Could you check a few things on this model? Use its own coordinates, in mm. Give positions to 0.01 mm unless a question says otherwise; leave off trailing zeros. Write each loop counter-clockwise with the first axis right and the second up, starting at its lowest first coordinate (ties: lowest second). Pieces come first, ordered by that corner, then holes. Notation, with made-up numbers: (-8.75, 9) - (13.25, 9) arc R21 cw to (13.25, 42) - close; hole circle Ø8 at (-13, -33.5). An arc over 180 degrees is marked (long way). Answer in a Markdown table with one row per item.
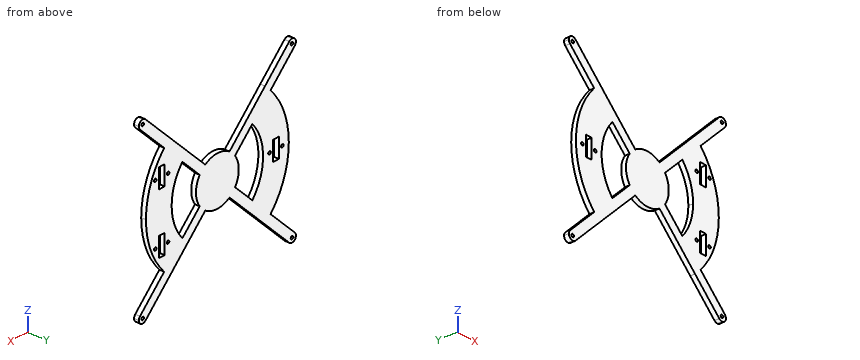
from build123d import *

# Parameters (mm, degrees)
SKETCH1_W           = 220
SKETCH1_H           = 220
SKETCH1_R           = 1.8
SKETCH1_W_2         = 8
SKETCH1_H_2         = 24
BOSS_EXTRUDE1_DEPTH = 3
CUT_EXTRUDE1_DEPTH  = 10


with BuildPart() as part:
    # Sketch1 → Boss-Extrude1 (new, symmetric)
    with BuildSketch(Plane(origin=(0, 0, 0), x_dir=(1, 0, 0), z_dir=(0, 1, 0))):
        Rectangle(SKETCH1_W, SKETCH1_H)
        with Locations(Location((-104.5, 104.5, 0), (0, 0, 270))):
            Circle(SKETCH1_R, mode=Mode.SUBTRACT)
        with Locations(Location((104.5, 104.5, 0), (0, 0, 90))):
            Circle(SKETCH1_R, mode=Mode.SUBTRACT)
        with Locations(Location((104.5, -104.5, 0), (0, 0, 270))):
            Circle(SKETCH1_R, mode=Mode.SUBTRACT)
        with Locations(Location((-104.5, -104.5, 0), (0, 0, 90))):
            Circle(SKETCH1_R, mode=Mode.SUBTRACT)
        with Locations(Location((-73, 0, 0), (0, 0, 270))):
            Circle(SKETCH1_R, mode=Mode.SUBTRACT)
        with Locations(Location((-91, 0, 0), (0, 0, 270))):
            Circle(SKETCH1_R, mode=Mode.SUBTRACT)
        with Locations(Location((87, 37, 0), (0, 0, 270))):
            Circle(SKETCH1_R, mode=Mode.SUBTRACT)
        with Locations(Location((69, 37, 0), (0, 0, 270))):
            Circle(SKETCH1_R, mode=Mode.SUBTRACT)
        with Locations(Location((87, -37, 0), (0, 0, 270))):
            Circle(SKETCH1_R, mode=Mode.SUBTRACT)
        with Locations(Location((69, -37, 0), (0, 0, 270))):
            Circle(SKETCH1_R, mode=Mode.SUBTRACT)
        with Locations((-82, 0)):
            Rectangle(SKETCH1_W_2, SKETCH1_H_2, mode=Mode.SUBTRACT)
        with Locations((78, 37)):
            Rectangle(SKETCH1_W_2, SKETCH1_H_2, mode=Mode.SUBTRACT)
        with Locations((78, -37)):
            Rectangle(SKETCH1_W_2, SKETCH1_H_2, mode=Mode.SUBTRACT)
    extrude(amount=BOSS_EXTRUDE1_DEPTH, both=True)

    # Sketch2 → Cut-Extrude1 (cut)
    with BuildSketch(Plane.XZ.offset(3)):
        with BuildLine():
            ThreePointArc((-108.389087297, 100.610912703), (-109.581337429, 102.395241122), (-110, 104.5))
            Line((-110, 104.5), (-110, -104.50000001))
            ThreePointArc((-110, -104.50000001), (-109.581337431, -102.395241127), (-108.389087297, -100.610912703))
            Line((-108.389087297, -100.610912703), (-74.492734511, -66.714559918))
            ThreePointArc((-74.492734511, -66.714559918), (-100, 0), (-74.492734511, 66.714559918))
            Line((-74.492734511, 66.714559918), (-108.389087297, 100.610912703))
        make_face()
        with BuildLine():
            Line((-24.74274405, 16.964569457), (-48.976502392, 41.198327799))
            ThreePointArc((-48.976502392, 41.198327799), (-64, 0), (-48.976502392, -41.198327799))
            Line((-48.976502392, -41.198327799), (-24.74274405, -16.964569457))
            ThreePointArc((-24.74274405, -16.964569457), (-30, 0), (-24.74274405, 16.964569457))
        make_face()
        with BuildLine():
            ThreePointArc((64, 0), (60.126933038, 21.926055812), (48.976502392, 41.198327799))
            Line((48.976502392, 41.198327799), (24.74274405, 16.964569457))
            ThreePointArc((24.74274405, 16.964569457), (28.65556073, 8.880249954), (30, 0))
            ThreePointArc((30, 0), (28.65556073, -8.880249954), (24.74274405, -16.964569457))
            Line((24.74274405, -16.964569457), (48.976502392, -41.198327799))
            ThreePointArc((48.976502392, -41.198327799), (60.126933038, -21.926055812), (64, 0))
        make_face()
        with BuildLine():
            Line((110, -104.5), (110, 104.5))
            ThreePointArc((110, 104.5), (109.581337429, 102.395241122), (108.389087297, 100.610912703))
            Line((108.389087297, 100.610912703), (74.492734511, 66.714559918))
            ThreePointArc((74.492734511, 66.714559918), (93.405763878, 35.71222864), (100, 0))
            ThreePointArc((100, 0), (93.405763878, -35.71222864), (74.492734511, -66.714559918))
            Line((74.492734511, -66.714559918), (108.389087297, -100.610912703))
            ThreePointArc((108.389087297, -100.610912703), (109.581337429, -102.395241122), (110, -104.5))
        make_face()
        with BuildLine():
            Line((-104.500000026, 110), (-110, 110))
            Line((-110, 110), (-110, 104.5))
            ThreePointArc((-110, 104.5), (-108.389087306, 108.389087287), (-104.500000026, 110))
        make_face()
        with BuildLine():
            ThreePointArc((-104.5, -110), (-108.389087293, -108.3890873), (-110, -104.50000001))
            Line((-110, -104.50000001), (-110, -110))
            Line((-110, -110), (-104.5, -110))
        make_face()
        with BuildLine():
            Line((110, -110), (110, -104.5))
            ThreePointArc((110, -104.5), (108.389087297, -108.389087297), (104.5, -110))
            Line((104.5, -110), (110, -110))
        make_face()
        with BuildLine():
            Line((110, 110), (104.5, 110))
            ThreePointArc((104.5, 110), (108.389087297, 108.389087297), (110, 104.5))
            Line((110, 104.5), (110, 110))
        make_face()
        with BuildLine():
            ThreePointArc((41.198327799, 48.976502392), (0, 64), (-41.198327799, 48.976502392))
            Line((-41.198327799, 48.976502392), (-16.964569457, 24.74274405))
            ThreePointArc((-16.964569457, 24.74274405), (0, 30), (16.964569457, 24.74274405))
            Line((16.964569457, 24.74274405), (41.198327799, 48.976502392))
        make_face()
        with BuildLine():
            ThreePointArc((66.714559918, 74.492734511), (0, 100), (-66.714559918, 74.492734511))
            Line((-66.714559918, 74.492734511), (-41.198327799, 48.976502392))
            ThreePointArc((-41.198327799, 48.976502392), (0, 64), (41.198327799, 48.976502392))
            Line((41.198327799, 48.976502392), (66.714559918, 74.492734511))
        make_face()
        with BuildLine():
            Line((104.5, 110), (-104.500000026, 110))
            ThreePointArc((-104.500000026, 110), (-102.395241134, 109.581337434), (-100.610912703, 108.389087297))
            Line((-100.610912703, 108.389087297), (-66.714559918, 74.492734511))
            ThreePointArc((-66.714559918, 74.492734511), (0, 100), (66.714559918, 74.492734511))
            Line((66.714559918, 74.492734511), (100.610912703, 108.389087297))
            ThreePointArc((100.610912703, 108.389087297), (102.395241122, 109.581337429), (104.5, 110))
        make_face()
        with BuildLine():
            ThreePointArc((-100.610912703, -108.389087297), (-102.395241122, -109.581337429), (-104.5, -110))
            Line((-104.5, -110), (104.5, -110))
            ThreePointArc((104.5, -110), (102.395241122, -109.581337429), (100.610912703, -108.389087297))
            Line((100.610912703, -108.389087297), (66.714559918, -74.492734511))
            ThreePointArc((66.714559918, -74.492734511), (0, -100), (-66.714559918, -74.492734511))
            Line((-66.714559918, -74.492734511), (-100.610912703, -108.389087297))
        make_face()
        with BuildLine():
            Line((-41.198327799, -48.976502392), (-66.714559918, -74.492734511))
            ThreePointArc((-66.714559918, -74.492734511), (0, -100), (66.714559918, -74.492734511))
            Line((66.714559918, -74.492734511), (41.198327799, -48.976502392))
            ThreePointArc((41.198327799, -48.976502392), (0, -64), (-41.198327799, -48.976502392))
        make_face()
        with BuildLine():
            Line((-16.964569457, -24.74274405), (-41.198327799, -48.976502392))
            ThreePointArc((-41.198327799, -48.976502392), (0, -64), (41.198327799, -48.976502392))
            Line((41.198327799, -48.976502392), (16.964569457, -24.74274405))
            ThreePointArc((16.964569457, -24.74274405), (0, -30), (-16.964569457, -24.74274405))
        make_face()
    extrude(amount=-CUT_EXTRUDE1_DEPTH, mode=Mode.SUBTRACT)


solid = part.part
1) Imagine slicing it at C-C (x = -14). List the corners of the cut face in (y, z) for me.
Check values:
| item | result |
|---|---|
| outline | (-3, -26.53) - (3, -26.53) - (3, 26.53) - (-3, 26.53) - close |
2) Imagine slicing it at A-A (x = 37.5). List the corners of the cut face in (y, z) for me.
Check values:
| item | result |
|---|---|
| outline | (-3, -45.28) - (3, -45.28) - (3, -29.72) - (-3, -29.72) - close; (-3, 29.72) - (3, 29.72) - (3, 45.28) - (-3, 45.28) - close |
3) If I drill on line 1 (X direction, y = 1.4, z = 0); line 2 (Z direction, x = 104.5, y = 1.3); line 3 (X direction, y = 2.2, z = 17), over which ranges is the centre line in solid material (lowest first)?
Check values:
| item | result |
|---|---|
| line 1 | x = -100 to -92.8, -89.2 to -86, -78 to -74.8, -71.2 to -64, -30 to 30, 64 to 100 |
| line 2 | z = -110 to -106.3, -102.7 to -96.72, 96.72 to 102.7, 106.3 to 110 |
| line 3 | x = -98.54 to -61.7, -24.78 to 24.78, 61.7 to 98.54 |
4) Will these pins go through, and if not, where does the flat tip stop? P1, Ø1, axis at y = 0, z = 74, coming from the +X side; P2, Ø3, axis at y = 1, z = -42, coming from the +X side; P3, Ø2, axis at y = -1, z = 60.5, coming from the +X side; P4, Ø3, axis at x = 104.5, z = 104.5, coming from the -Y side.
Check values:
| item | result |
|---|---|
| P1 | stops at x = 82.28 |
| P2 | stops at x = 91.43 |
| P3 | stops at x = 80.37 |
| P4 | passes through |
5) Imagine slicing it at B-B (y = -0.7). State how many separate pieces and enclosed holes the cut face has, then the cut area to 3 significant figures.
Check values:
| item | result |
|---|---|
| separate pieces | 1 |
| enclosed holes | 15 |
| area | 16,000 mm2 |
